Part model, mm, in its own coordinate system. Face numbers are marked on the shaded views. A direction names the side the tool comes from. Give positions to 0.01 mm unless a question says otherwise; leave off trailing zeros. Write each loop counter-clockwise with the first axis right and the second up, starting at its lowest first coordinate (ties: lowest second). Pieces come first, ordered by that corner, then holes. Notation, with made-up numbers: M -35.75,44 L 8.25,44 A12 ccw 8.25,49 Z; hole C -5.5,40.25 d6. An arc over 180 degrees is marked long. Use a Markdown table: item, result.
```python
from build123d import *

# Parameters (mm, degrees)
SKETCH2_W               = 42
SKETCH2_H               = 40
BOSS_EXTRUDE1_DEPTH     = 12.15
CUT_EXTRUDE1_DEPTH      = 149.231651478
CUT_EXTRUDE1_DEPTH_BACK = 149.231651478
SKETCH3_R               = 3.25
FILLET1_R               = 25
FILLET2_R               = 5
SKETCH4_R               = 3.9
BOSS_EXTRUDE2_DEPTH     = 2.8
CHAMFER1_SIZE           = 0.5
SKETCH6_W               = 20
SKETCH6_H               = 11.3
BOSS_EXTRUDE3_DEPTH     = 22
BOSS_EXTRUDE5_DEPTH     = 12
SKETCH7_R               = 2.65
CUT_EXTRUDE2_DEPTH      = 10
FILLET3_R               = 10
CHAMFER3_SIZE           = 2
SKETCH9_R               = 3.25
CUT_EXTRUDE3_DEPTH      = 2


# Some blends are built 0.0001 mm under size
with BuildPart() as part:
    # Sketch2 → Boss-Extrude1 (new, symmetric)
    with BuildSketch(Plane.XY):
        Polygon((-33, 0), (33, 0), (33, -144), (21, -144), (21, -99), (-21, -99), (-21, -144), (-33, -144), align=None)
        with Locations((0, -32)):
            Rectangle(SKETCH2_W, SKETCH2_H, mode=Mode.SUBTRACT)
        with Locations((0, -75.5)):
            Rectangle(SKETCH2_W, SKETCH2_H, mode=Mode.SUBTRACT)
    extrude(amount=BOSS_EXTRUDE1_DEPTH, both=True)

    # Sketch3 → Cut-Extrude1 (cut, two sides: drawn at the far end of the back side and taken through both)
    with BuildSketch(Plane(origin=(0, 0, 0), x_dir=(0, 0, -1), z_dir=(1, 0, 0)).offset(-CUT_EXTRUDE1_DEPTH_BACK)):
        with Locations((0, -106)):
            Circle(SKETCH3_R)
        with Locations((0, -62.5)):
            Circle(SKETCH3_R)
        with Locations((0, -19)):
            Circle(SKETCH3_R)
        with Locations((6, -136)):
            Circle(SKETCH3_R)
    extrude(amount=CUT_EXTRUDE1_DEPTH + CUT_EXTRUDE1_DEPTH_BACK, mode=Mode.SUBTRACT)

    # Fillet1
    # the kernel refuses this fillet: 25 mm, written as the material it takes off along each edge
    with BuildSketch(Plane(origin=(95.475495196, -144, 12.15), x_dir=(0, 1, 0), z_dir=(-1, 0, 0)), Plane(origin=(41.475495196, -144, 12.15), x_dir=(0, 1, 0), z_dir=(-1, 0, 0))) as fillet1_piece_1:
        with BuildLine():
            CenterArc((24.990198078, 25), FILLET1_R, 181.604491527, 88.395508473)
            Line((0, 24.3), (-0.499803962, 24.286))
            ThreePointArc((-0.499803962, 24.286), (-0.5, 12.15), (-0.5, 0))
            Line((-0.5, 0), (0, -0.5))
            Line((0, -0.5), (24.990198078, -0.5))
            Line((24.990198078, -0.5), (24.990198078, 0))
        make_face()
    extrude(amount=136.950990392, mode=Mode.SUBTRACT)

    # Fillet2
    fillet2_edges = [part.edges().sort_by_distance(p)[0] for p in [
        (-27, -144, -12.15),
        (27, -144, -12.15),
    ]]
    fillet(fillet2_edges, radius=FILLET2_R)

    # Sketch4 → Boss-Extrude2 (add)
    with BuildSketch(Plane(origin=(0, 0, 12.15), x_dir=(-1, 0, 0), z_dir=(0, 0, -1))):
        with Locations((-27, -6)):
            Circle(SKETCH4_R)
        with Locations((27, -6)):
            Circle(SKETCH4_R)
        with Locations((27, -106)):
            Circle(SKETCH4_R)
        with Locations((-27, -106)):
            Circle(SKETCH4_R)
    extrude(amount=-BOSS_EXTRUDE2_DEPTH)

    # Chamfer1
    chamfer1_edges = [part.edges().sort_by_distance(p)[0] for p in [
        (30.9, -6, 14.95),
        (-23.1, -6, 14.95),
        (-23.1, -106, 14.95),
        (30.9, -106, 14.95),
    ]]
    chamfer(chamfer1_edges, length=CHAMFER1_SIZE)

    # Sketch6 → Boss-Extrude3 (add)
    with BuildSketch(Plane(origin=(55, 0, 0), x_dir=(0, 0, -1), z_dir=(1, 0, 0))):
        with Locations((0, -26.54)):
            Rectangle(SKETCH6_W, SKETCH6_H)
        with Locations((0, -78.24)):
            Rectangle(SKETCH6_W, SKETCH6_H)
        Polygon((-1.125133679, -148.289856389), (18.225525462, -143.234958685), (21.081542665, -154.168081099), (1.730883524, -159.222978804), align=None)
        Polygon((-11.336027041, -97.522336202), (5.158614897, -93.213504805), (8.0146321, -104.146627219), (-11.336027041, -109.201524924), align=None)
    extrude(amount=-BOSS_EXTRUDE3_DEPTH)


with BuildPart() as boss_extrude3_piece_1:
    # of the separate pieces the step leaves, piece 1, a body of its own (boss_extrude3_pieces)
    add(part.part.solids().sort_by_distance((23.1, -106, 14.45))[0])



with BuildPart() as boss_extrude3_piece_2:
    # of the separate pieces the step leaves, piece 2, a body of its own (boss_extrude3_pieces)
    add(part.part.solids().sort_by_distance((55, -148.289856389, 1.125133679))[0])


with BuildPart() as boss_extrude3_piece_1_1:
    add(boss_extrude3_piece_1.part)

    add(boss_extrude3_piece_2.part)  # Boss-Extrude5 merges Boss-Extrude3 piece 2
    # Sketch8 → Boss-Extrude5 (add)
    with BuildSketch(Plane(origin=(33, 0, 0), x_dir=(0, 0, -1), z_dir=(1, 0, 0))):
        with BuildLine():
            Line((-1.125133679, -148.289856389), (-3.933707562, -137.538351797))
            ThreePointArc((-3.933707562, -137.538351797), (0.590701612, -140.797633457), (5.725, -142.972989836))
            ThreePointArc((5.725, -142.972989836), (10.139565186, -142.188157138), (12.15, -138.180352253))
            Line((12.15, -138.180352253), (12.15, -119.977233364))
            Line((12.15, -119.977233364), (18.225525462, -143.234958685))
            Line((18.225525462, -143.234958685), (21.081542665, -154.168081099))
            Line((21.081542665, -154.168081099), (1.730883524, -159.222978804))
            Line((1.730883524, -159.222978804), (-1.125133679, -148.289856389))
        make_face()
    extrude(amount=-BOSS_EXTRUDE5_DEPTH)

    # Sketch7 → Cut-Extrude2 (cut)
    with BuildSketch(Plane(origin=(55, 0, 0), x_dir=(0, 0, -1), z_dir=(1, 0, 0))):
        with Locations((-4.75, -27.89)):
            Circle(SKETCH7_R)
        with Locations((4.75, -27.89)):
            Circle(SKETCH7_R)
        with Locations((-4.75, -76.89)):
            Circle(SKETCH7_R)
        with Locations((4.75, -76.89)):
            Circle(SKETCH7_R)
        with Locations((-7.343282023, -103.714222561)):
            Circle(SKETCH7_R)
        with Locations((1.848281069, -101.313146151)):
            Circle(SKETCH7_R)
        with Locations((5.041217352, -151.123337457)):
            Circle(SKETCH7_R)
        with Locations((14.232780444, -148.722261047)):
            Circle(SKETCH7_R)
    extrude(amount=-CUT_EXTRUDE2_DEPTH, mode=Mode.SUBTRACT)

    # Fillet3
    fillet3_edges = [boss_extrude3_piece_1_1.edges().sort_by_distance(p)[0] for p in [
        (38, -159.222978804, -1.730883524),
        (38, -154.168081099, -21.081542665),
        (27, -119.977233364, -12.15),
        (27, -137.538351797, 3.933707562),
    ]]
    fillet(fillet3_edges, radius=FILLET3_R - 0.0001)  # a hair under: the kernel refuses the full size

    # Chamfer3
    # the kernel refuses this chamfer: 2 mm, written as the material it adds along each edge
    with BuildSketch(Plane(origin=(33, -20.89, 2.499429517), x_dir=(-0.027495876610585647, 0.9996219169112968, 0), z_dir=(0, 0, -1))) as chamfer3_piece_1_section:
        Polygon((CHAMFER3_SIZE * 0.999621916911, CHAMFER3_SIZE * 0.0274958766106), (-CHAMFER3_SIZE * 0.0274958766106, CHAMFER3_SIZE * 0.999621916911), (0, 0), align=None)
    chamfer3_piece_1 = extrude(amount=12.499429517, mode=Mode.PRIVATE)
    chamfer3_piece_1 = chamfer3_piece_1 - Plane(origin=(33.672455273, -19, 0), x_dir=(0, 0, -1), z_dir=(-1, 0, 0)) * Cylinder(3.25, 33, mode=Mode.PRIVATE)
    add(chamfer3_piece_1)
    with BuildSketch(Plane(origin=(33, -20.89, 10), x_dir=(-0.027495876610585647, 0.9996219169112968, 0), z_dir=(0, 0, -1))) as chamfer3_piece_2_section:
        Polygon((CHAMFER3_SIZE * 0.999621916911, CHAMFER3_SIZE * 0.0274958766106), (-CHAMFER3_SIZE * 0.0274958766106, CHAMFER3_SIZE * 0.999621916911), (0, 0), align=None)
    chamfer3_piece_2 = extrude(amount=12.499429517, mode=Mode.PRIVATE)
    chamfer3_piece_2 = chamfer3_piece_2 - Plane(origin=(33.672455268, -19, 0), x_dir=(0, 0, -1), z_dir=(-1, 0, 0)) * Cylinder(3.25, 33, mode=Mode.PRIVATE)
    add(chamfer3_piece_2)
    with BuildSketch(Plane(origin=(33, -32.19, -10), x_dir=(-0.027495876610585647, -0.9996219169112968, 0), z_dir=(0, 0, 1)), Plane(origin=(33, -72.59, 10), x_dir=(-0.02749587661058555, 0.9996219169112968, 0), z_dir=(0, 0, -1)), Plane(origin=(33, -83.89, -10), x_dir=(-0.02749587661058555, -0.9996219169112968, 0), z_dir=(0, 0, 1)), Plane(origin=(33, -148.289856389, 1.125133679), x_dir=(-0.02749587661058553, 0.967167149212802, 0.2526493266426751), z_dir=(0, 0.25274488520952904, -0.96753295706163))) as chamfer3_piece_3:
        Polygon((CHAMFER3_SIZE * 0.999621916911, CHAMFER3_SIZE * 0.0274958766106), (-CHAMFER3_SIZE * 0.0274958766106, CHAMFER3_SIZE * 0.999621916911), (0, 0), align=None)
    extrude(amount=20)
    with BuildSketch(Plane(origin=(33, -105.744268383, -1.898700305), x_dir=(-0.0274958766105857, -0.9671671492128014, -0.25264932664267675), z_dir=(0, -0.25274488520953076, 0.9675329570616297))) as chamfer3_piece_4_section:
        Polygon((CHAMFER3_SIZE * 0.999621916911, CHAMFER3_SIZE * 0.0274958766106), (-CHAMFER3_SIZE * 0.0274958766106, CHAMFER3_SIZE * 0.999621916911), (0, 0), align=None)
    chamfer3_piece_4 = extrude(amount=18.822204769, mode=Mode.PRIVATE)
    chamfer3_piece_4 = chamfer3_piece_4 - Plane(origin=(33.659062182, -106, 0), x_dir=(0, 0, -1), z_dir=(-1, 0, 0)) * Cylinder(3.25, 46, mode=Mode.PRIVATE)
    chamfer3_piece_4 = split(chamfer3_piece_4, bisect_by=Plane(origin=(33.659062182, -108.784347248, 11.336027041), z_dir=(0, 0, -1)), keep=Keep.TOP, mode=Mode.PRIVATE)
    add(chamfer3_piece_4)
    with BuildSketch(Plane(origin=(33, -98.822295645, 16.312403133), x_dir=(-0.027495876610585716, 0.9671671492128022, 0.25264932664267414), z_dir=(0, 0.25274488520952815, -0.9675329570616303))) as chamfer3_piece_5_section:
        Polygon((CHAMFER3_SIZE * 0.999621916911, CHAMFER3_SIZE * 0.0274958766106), (-CHAMFER3_SIZE * 0.0274958766106, CHAMFER3_SIZE * 0.999621916911), (0, 0), align=None)
    chamfer3_piece_5 = extrude(amount=22.191510763, mode=Mode.PRIVATE)
    chamfer3_piece_5 = split(chamfer3_piece_5, bisect_by=Plane(origin=(33.668386777, -94.70433277, 11.336027041), z_dir=(0, 0, -1)), keep=Keep.TOP, mode=Mode.PRIVATE)
    add(chamfer3_piece_5)
    with BuildSketch(Plane(origin=(33, -104.146627219, -8.0146321), x_dir=(-0.027495876610585706, -0.9671671492128016, -0.25264932664267675), z_dir=(0, -0.25274488520953076, 0.9675329570616297))) as chamfer3_piece_6_section:
        Polygon((CHAMFER3_SIZE * 0.999621916911, CHAMFER3_SIZE * 0.0274958766106), (-CHAMFER3_SIZE * 0.0274958766106, CHAMFER3_SIZE * 0.999621916911), (0, 0), align=None)
    chamfer3_piece_6 = extrude(amount=10.124541165, mode=Mode.PRIVATE)
    chamfer3_piece_6 = chamfer3_piece_6 - Plane(origin=(33.659192964, -106, 0), x_dir=(0, 0, -1), z_dir=(-1, 0, 0)) * Cylinder(3.25, 29, mode=Mode.PRIVATE)
    add(chamfer3_piece_6)

    # Sketch9 → Cut-Extrude3 (cut)
    with BuildSketch(Plane(origin=(33, 0, 0), x_dir=(0, 0, -1), z_dir=(1, 0, 0))):
        with Locations((0, -19)):
            Circle(SKETCH9_R)
        with Locations((0, -106)):
            Circle(SKETCH9_R)
    extrude(amount=CUT_EXTRUDE3_DEPTH, mode=Mode.SUBTRACT)


solid = boss_extrude3_piece_1_1.part
```
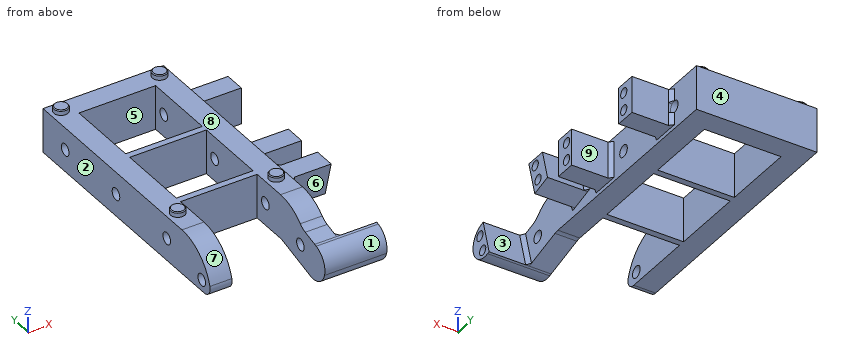
1. Drill centre lines: L1, parallel to Y at x = -6, z = 9.5; L2, parallel to X at y = -86.5, z = 1; L3, parallel to X at y = -93.5, z = -2. Where is each one in solid material? Low to high.
Findings below:
| item | result |
|---|---|
| L1 | -99 to -95.5, -55.5 to -52, -12 to 0 |
| L2 | -33 to -21, 21 to 33 |
| L3 | -33 to -21, 21 to 34.48 |
2. Cut at C-C, the plane y = -6. Give the cut face in (x, z), then the cut area to 3 significant figures.
Findings below:
| item | result |
|---|---|
| outline | M -33,-12.15 L 33,-12.15 L 33,12.15 L 30.9,12.15 L 30.9,14.45 L 30.4,14.95 L 23.6,14.95 L 23.1,14.45 L 23.1,12.15 L -23.1,12.15 L -23.1,14.45 L -23.6,14.95 L -30.4,14.95 L -30.9,14.45 L -30.9,12.15 L -33,12.15 Z |
| area | 1,650 mm2 |
3. Two-plate mould, pull along Y, no slides. Class the marked faces 1, 2, 3 and 4: released by +Y, released by -Y, zero draft, split by the parting line, or undercut.
Findings below:
| item | result |
|---|---|
| face 1 | released by -Y |
| face 2 | zero draft |
| face 3 | undercut |
| face 4 | released by +Y |
4. Tool access for the marked faces 5, 6, 7, 8 and 9: list every direction of +Z, -Z, +X, -X, +Y, -Y with a clear straight run to the whole face (end or side of a thin tool).
Findings below:
| item | result |
|---|---|
| face 5 | +Z, -Z |
| face 6 | -Z, +X |
| face 7 | +Z, -X, -Y |
| face 8 | +Z |
| face 9 | +Z, -Z, +X |
5. Drop flat-ended pins along their axis: P1, Ø7.5, axis at x = -1.5, z = 5, coming from the -Y side; P2, Ø7.5, axis at y = -128, z = 3, coming from the +X side; P3, Ø2.5, axis at y = -77.5, z = 5.5, coming from the +X side. Give the stop position or say it passes through.
Findings below:
| item | result |
|---|---|
| P1 | y = -99 |
| P2 | x = 33 |
| P3 | x = 45 |
6. Cut at A-A, the plane x = -8.5. Give the cut face in (y, z), then the cut area to 3 significant figures.
Findings below:
| item | result |
|---|---|
| outline | M -99,-12.15 L -95.5,-12.15 L -95.5,12.15 L -99,12.15 Z; M -55.5,-12.15 L -52,-12.15 L -52,12.15 L -55.5,12.15 Z; M -12,-12.15 L 0,-12.15 L 0,12.15 L -12,12.15 Z |
| area | 462 mm2 |
7. Cut at B-B, the plane y = -76.89. Give the cut face in (x, z), then the cut area to 3 significant figures.
Findings below:
| item | result |
|---|---|
| outline | M -33,-12.15 L -21,-12.15 L -21,12.15 L -33,12.15 Z; M 21,-12.15 L 33,-12.15 L 33,-10 L 55,-10 L 55,-7.4 L 45,-7.4 L 45,-2.1 L 55,-2.1 L 55,2.1 L 45,2.1 L 45,7.4 L 55,7.4 L 55,10 L 33,10 L 33,12.15 L 21,12.15 Z |
| area | 917 mm2 |
